Geometry check sheet. Reference: the model listing, model coordinates, mm. Round coordinates to 2 decimals unless told otherwise and drop trailing zeros. Write each loop counter-clockwise with the first axis right and the second up, starting at its lowest first coordinate (ties: lowest second). Pieces come first, ordered by that corner, then holes.
Item 1: Cross-section at A-A (y = 3.15). State how many separate pieces and enclosed holes the cut face has, then the cut area to 3 significant figures.
Item 2: Cross-section at C-C (z = 63). Enter the section's corners in (x, y), then the cut area to 3 significant figures.
Item 3: Depth check by flat-ended pin: P1, Ø1.5, axis at y = 3, z = -214.5, coming from the -X side. Enter the tip coordinate at first touch or a pass-through.
Item 4: Scan lines: probe 1 along Z at (x, y) = (8.5, 1.5); probe 2 along X at (y, z) = (1, -248.5); probe 3 along X at (y, z) = (1.1, -142). Record each from-to range of solid material in increasing order.
Item 5: Cross-section at B-B (x = -87). Enter the section's corners in (y, z).
from build123d import *

# Parameters (mm, degrees)
SKETCH1_R           = 309.88
BOSS_EXTRUDE1_DEPTH = 5.842
SKETCH2_R           = 2.5527
CUT_EXTRUDE1_DEPTH  = 439.275435958
CIRPATTERN1_COUNT   = 9
SKETCH3_R           = 2.5527
HOLE_WIRE_DEPTH     = 439.275435958


with BuildPart() as part:
    # Sketch1 → Boss-Extrude1 (new body)
    with BuildSketch(Plane(origin=(0, 0, 0), x_dir=(1, 0, 0), z_dir=(0, 1, 0))):
        with Locations(Location((0, 0, 0), (0, 0, 270))):
            Circle(SKETCH1_R)
    extrude(amount=BOSS_EXTRUDE1_DEPTH)

    # Sketch2 → Cut-Extrude1 (cut, through all)
    with BuildSketch(Plane(origin=(0, 5.842, 0), x_dir=(1, 0, 0), z_dir=(0, 1, 0))):
        with Locations(Location((-290.734014455, 77.901944385, 0), (0, 0, 270))):
            Circle(SKETCH2_R)
        with Locations(Location((-290.734014455, -77.901944385, 0), (0, 0, 270))):
            Circle(SKETCH2_R)
    cut_extrude1 = extrude(amount=-CUT_EXTRUDE1_DEPTH, mode=Mode.SUBTRACT)

    # CirPattern1: Cut-Extrude1 ×9 about axis
    cirpattern1_axis = Axis((0, 0, 0), (0, 1, 0))
    for i in range(1, CIRPATTERN1_COUNT):
        add(cut_extrude1.rotate(cirpattern1_axis, i * 360 / CIRPATTERN1_COUNT), mode=Mode.SUBTRACT)

    # Sketch3 → Hole_Wire (cut, through all)
    with BuildSketch(Plane(origin=(0, 5.842, 0), x_dir=(1, 0, 0), z_dir=(0, 1, 0))):
        with Locations(Location((260.664986285, 150.495, 0), (0, 0, 270))):
            Circle(SKETCH3_R)
    extrude(amount=-HOLE_WIRE_DEPTH, mode=Mode.SUBTRACT)


solid = part.part
Resolved:
1. separate pieces: 1
1. enclosed holes: 19
1. area: 301,000 mm2
2. outline: (-303.41, 0) - (303.41, 0) - (303.41, 5.84) - (-303.41, 5.84) - close
2. area: 3,550 mm2
3. P1: stops at x = -224.36
4. probe 1: z = -309.76 to 309.76
4. probe 2: x = -185.13 to -174.3, -170.99 to 185.13
4. probe 3: x = -275.43 to 275.43
5. outline: (0, -297.42) - (5.84, -297.42) - (5.84, 297.42) - (0, 297.42) - close
